CAD build for the part. Positions are in the model's coordinates, mm. A direction names the side the tool comes from. Give positions to 0.01 mm unless a question says otherwise; leave off trailing zeros. Order: outer loops, then holes, each group sorted by start corner. A loop starts at its lowest first (then second) coordinate and runs counter-clockwise, first axis right, second up.
from build123d import *

# Parameters (mm, degrees)
SKETCH1_W            = 18
SKETCH1_H            = 18.5
BOSS_EXTRUDE1_DEPTH  = 3.3
SKETCH2_W            = 18
SKETCH2_H            = 18.5
BOSS_EXTRUDE2_DEPTH  = 0.7
FILLET1_R            = 3
SKETCH3_W            = 13.9
SKETCH3_H            = 14.6
BOSS_EXTRUDE3_DEPTH  = 3.9
SKETCH4_W            = 13.9
SKETCH4_H            = 14.6
SKETCH4_R            = 4.25
BOSS_EXTRUDE4_DEPTH  = 1.5
CHAMFER1_SIZE        = 1
BOSS_EXTRUDE5_DEPTH  = 2
SKETCH6_W            = 0.6
SKETCH6_H            = 6
CUT_EXTRUDE1_DEPTH   = 15.876911642
SKETCH7_W            = 0.7
SKETCH7_H            = 6
CUT_EXTRUDE2_DEPTH   = 14
SKETCH8_W            = 2.65
SKETCH8_H            = 2.4
BOSS_EXTRUDE6_DEPTH  = 0.2
SKETCH9_W            = 2.65
SKETCH9_H            = 2.4
BOSS_EXTRUDE7_DEPTH  = 0.2
CUT_EXTRUDE3_DEPTH   = 18.893085257
CUT_EXTRUDE5_START   = -7.9
CUT_EXTRUDE5_DEPTH   = 7.9
CUT_EXTRUDE7_START   = -4.6
SKETCH12_W           = 0.378675411
SKETCH12_H           = 6.25
CUT_EXTRUDE7_DEPTH   = 4.6
BOSS_EXTRUDE10_DEPTH = 3.3
FILLET2_R            = 2
BOSS_EXTRUDE11_DEPTH = 0.6
SKETCH15_R           = 1.3
CUT_EXTRUDE8_DEPTH   = 18.622783549


with BuildPart() as part:
    # Sketch1 → Boss-Extrude1 (new body)
    with BuildSketch(Plane.XY):
        Rectangle(SKETCH1_W, SKETCH1_H)
        Polygon((-3, -8.25), (-3, -3.25), (-8.2, -3.25), (-8.2, 8.25), (3, 8.25), (3, 3.25), (7.473843231, 3.25), (8.2, 3.25), (8.2, -8.25), align=None, mode=Mode.SUBTRACT)
    extrude(amount=BOSS_EXTRUDE1_DEPTH)

    # Sketch2 → Boss-Extrude2 (add)
    with BuildSketch(Plane.XY.offset(3.3)):
        Rectangle(SKETCH2_W, SKETCH2_H)
        Polygon((-6, 6.5), (3, 6.5), (3, 3.25), (6, 3.25), (6, -6.5), (-3, -6.5), (-3, -3.25), (-6, -3.25), align=None, mode=Mode.SUBTRACT)
    extrude(amount=BOSS_EXTRUDE2_DEPTH)

    # Fillet1
    fillet1_edges = [part.edges().sort_by_distance(p)[0] for p in [
        (-9, 9.25, 2),
        (9, 9.25, 2),
        (9, -9.25, 2),
        (-9, -9.25, 2),
    ]]
    fillet(fillet1_edges, radius=FILLET1_R)

    # Sketch3 → Boss-Extrude3 (add)
    with BuildSketch(Plane.XY.offset(4)):
        Rectangle(SKETCH3_W, SKETCH3_H)
        Polygon((-6, 6.5), (3, 6.5), (3, 3.25), (6, 3.25), (6, -6.5), (-3, -6.5), (-3, -3.25), (-6, -3.25), align=None, mode=Mode.SUBTRACT)
    extrude(amount=BOSS_EXTRUDE3_DEPTH)

    # Sketch4 → Boss-Extrude4 (add)
    with BuildSketch(Plane.XY.offset(7.9)):
        Rectangle(SKETCH4_W, SKETCH4_H)
        Circle(SKETCH4_R, mode=Mode.SUBTRACT)
    extrude(amount=BOSS_EXTRUDE4_DEPTH)

    # Chamfer1
    chamfer1_edges = [part.edges().sort_by_distance(p)[0] for p in [
        (-6.95, 7.3, 6.7),
        (-6.95, -7.3, 6.7),
        (6.95, -7.3, 6.7),
        (6.95, 7.3, 6.7),
        (-6.95, 0, 9.4),
        (0, -7.3, 9.4),
        (6.95, 0, 9.4),
        (0, 7.3, 9.4),
    ]]
    chamfer(chamfer1_edges, length=CHAMFER1_SIZE)

    # Sketch5 → Boss-Extrude5 (add)
    with BuildSketch(Plane.XY.offset(9.4)):
        with BuildLine():
            Line((-2.846728769, 4.470585567), (-2.109207508, 3.689680703))
            ThreePointArc((-2.109207508, 3.689680703), (3.089805898, 2.918150015), (3.563233813, -2.316433637))
            Line((3.563233813, -2.316433637), (4.300755074, -3.097338502))
            ThreePointArc((4.300755074, -3.097338502), (3.853169709, 3.639104725), (-2.846728769, 4.470585567))
        make_face()
        with BuildLine():
            Line((2.846728769, -4.470585567), (2.109207508, -3.689680703))
            ThreePointArc((2.109207508, -3.689680703), (-3.089805898, -2.918150015), (-3.563233813, 2.316433637))
            Line((-3.563233813, 2.316433637), (-4.300755074, 3.097338502))
            ThreePointArc((-4.300755074, 3.097338502), (-3.853169709, -3.639104725), (2.846728769, -4.470585567))
        make_face()
    extrude(amount=BOSS_EXTRUDE5_DEPTH)

    # Sketch6 → Cut-Extrude1 (cut, through all)
    with BuildSketch(Plane.XY.offset(4)):
        with Locations((7.25, 0)):
            Rectangle(SKETCH6_W, SKETCH6_H)
        with Locations((-7.25, 0)):
            Rectangle(SKETCH6_W, SKETCH6_H)
    extrude(amount=-CUT_EXTRUDE1_DEPTH, mode=Mode.SUBTRACT)

    # Sketch7 → Cut-Extrude2 (cut)
    with BuildSketch(Plane(origin=(6.95, 0, 0), x_dir=(0, 0, -1), z_dir=(1, 0, 0))):
        with Locations((-3.65, 0)):
            Rectangle(SKETCH7_W, SKETCH7_H)
    extrude(amount=-CUT_EXTRUDE2_DEPTH, mode=Mode.SUBTRACT)

    # Sketch8 → Boss-Extrude6 (add)
    with BuildSketch(Plane(origin=(6.95, 0, 0), x_dir=(0, 0, -1), z_dir=(1, 0, 0))):
        with Locations((-6.575, 0)):
            Rectangle(SKETCH8_W, SKETCH8_H)
    extrude(amount=BOSS_EXTRUDE6_DEPTH)

    # Sketch9 → Boss-Extrude7 (add)
    with BuildSketch(Plane.ZY.offset(6.95)):
        with Locations((6.575, 0)):
            Rectangle(SKETCH9_W, SKETCH9_H)
    extrude(amount=BOSS_EXTRUDE7_DEPTH)

    # Sketch10 → Cut-Extrude3 (cut, through all)
    with BuildSketch(Plane.XZ.offset(1.2)):
        Polygon((-6.95, 7.9), (-7.15, 5.85), (-7.15, 7.9), align=None)
        Polygon((6.95, 7.9), (7.15, 5.85), (7.15, 7.9), align=None)
    extrude(amount=-CUT_EXTRUDE3_DEPTH, mode=Mode.SUBTRACT)

    # Sketch11 → Cut-Extrude5 (cut)
    with BuildSketch(Plane(origin=(0, 0, 0), x_dir=(-1, 0, 0), z_dir=(0, 0, -1)).offset(CUT_EXTRUDE5_START)):
        with BuildLine():
            Line((-4.578389967, 6.802818924), (-3.862648789, 6.027432648))
            ThreePointArc((-3.862648789, 6.027432648), (-3.439450113, 6.278549428), (-3, 6.5))
            Line((-3, 6.5), (-3, 3.25))
            Line((-3, 3.25), (-6.378675411, 3.25))
            ThreePointArc((-6.378675411, 3.25), (-6.063337952, 3.806039001), (-5.699657401, 4.331732391))
            Line((-5.699657401, 4.331732391), (-6.415398578, 5.107118667))
            ThreePointArc((-6.415398578, 5.107118667), (-5.290584801, 5.731466868), (-4.578389967, 6.802818924))
        make_face()
        with BuildLine():
            Line((4.578389967, -6.802818924), (3.862648789, -6.027432648))
            ThreePointArc((3.862648789, -6.027432648), (3.439450113, -6.278549428), (3, -6.5))
            Line((3, -6.5), (3, -3.25))
            Line((3, -3.25), (6.378675411, -3.25))
            ThreePointArc((6.378675411, -3.25), (6.063337952, -3.806039001), (5.699657401, -4.331732391))
            Line((5.699657401, -4.331732391), (6.415398578, -5.107118667))
            ThreePointArc((6.415398578, -5.107118667), (5.290584801, -5.731466868), (4.578389967, -6.802818924))
        make_face()
    extrude(amount=CUT_EXTRUDE5_DEPTH, mode=Mode.SUBTRACT)

    # Sketch12 → Cut-Extrude7 (cut)
    with BuildSketch(Plane(origin=(0, 0, 3.3), x_dir=(-1, 0, 0), z_dir=(0, 0, -1)).offset(CUT_EXTRUDE7_START)):
        with Locations((-6.189337705, 0.125)):
            Rectangle(SKETCH12_W, SKETCH12_H)
        with Locations((6.189337705, -0.125)):
            Rectangle(SKETCH12_W, SKETCH12_H)
    extrude(amount=CUT_EXTRUDE7_DEPTH, mode=Mode.SUBTRACT)

    # Sketch13 → Boss-Extrude10 (add)
    with BuildSketch(Plane(origin=(0, 0, 0), x_dir=(-1, 0, 0), z_dir=(0, 0, -1))):
        with BuildLine():
            Line((-1.342004098, -8.25), (1.342004098, -8.25))
            ThreePointArc((1.342004098, -8.25), (0, -7.69645725), (-1.342004098, -8.25))
        make_face()
        with BuildLine():
            Line((-1.342004098, 8.25), (1.342004098, 8.25))
            ThreePointArc((1.342004098, 8.25), (0, 7.695), (-1.342004098, 8.25))
        make_face()
    extrude(amount=-BOSS_EXTRUDE10_DEPTH)

    # Fillet2
    fillet2_edges = [part.edges().sort_by_distance(p)[0] for p in [
        (-8.2, 8.25, 1.65),
        (8.2, -8.25, 1.65),
    ]]
    fillet(fillet2_edges, radius=FILLET2_R)

    # Sketch14 → Boss-Extrude11 (add)
    with BuildSketch(Plane(origin=(0, 0, 0), x_dir=(-1, 0, 0), z_dir=(0, 0, -1))):
        with BuildLine():
            Line((-1.871089255, -9.25), (1.871089255, -9.25))
            ThreePointArc((1.871089255, -9.25), (0, -7.69645725), (-1.871089255, -9.25))
        make_face()
        with BuildLine():
            Line((-1.871089255, 9.25), (1.871089255, 9.25))
            ThreePointArc((1.871089255, 9.25), (0, 7.69645725), (-1.871089255, 9.25))
        make_face()
    extrude(amount=BOSS_EXTRUDE11_DEPTH)

    # Sketch15 → Cut-Extrude8 (cut, through all)
    with BuildSketch(Plane(origin=(0, 0, -0.6), x_dir=(-1, 0, 0), z_dir=(0, 0, -1))):
        with Locations((0, 9.6)):
            Circle(SKETCH15_R)
        with Locations((0, -9.6)):
            Circle(SKETCH15_R)
    extrude(amount=-CUT_EXTRUDE8_DEPTH, mode=Mode.SUBTRACT)


solid = part.part
1. Saw through at B-B on y = 1.5. State how many separate pieces and enclosed holes the cut face has, plus the area to 3 significant figures.
2. Pin check, flat tips, straight feed: P1, Ø5.5, axis at x = 3, y = -0.5, coming from the -Z side; P2, Ø0.6, axis at x = 6.5, y = -1.5, coming from the -Z side; P3, Ø0.8, axis at x = -6.5, z = 4.5, coming from the -Y side. Stop position of each tip, or through.
3. Saw through at D-D on y = -4. Give the cut face in (x, z), plus the area to 3 significant figures.
4. Mould opens along X. For faces 4 (the flat face through (5, -7, 3.3)), 5 (the flat face through (-6.27, -6.6, 8.78)), 6 (the cylindrical face through (-7.63, 7.65, 1.67)), 7 (the flat face through (6.44, -0.09, 8.91)) say: released by +X, released by -X, zero draft, split by the parting line, or undercut.
5. 3-axis set-ups, long thin cutter, end or side, ignore diameter. For faces 1 (the flat face through (-6.44, 6.81, 6.23)), 2 (the cylindrical face through (3.923, 3.564, 10.386)), 3 (the flat face through (-4, 8.25, 2)): which of +Z, -Z, +X, -X, +Y, -Y reach the whole face in a straight line?
6. Wall check: line 1 (Y direction, x = 0.25, z = 7); line 2 (X direction, y = 0, z = 8.35); line 3 (Z direction, x = -0.75, y = -5.5). Give the ranges that are in metal, low to high.
7. Saw through at C-C on z = 4.5. Give the cut face in (x, y), plus the area to 3 significant figures.
Reported:
1. separate pieces: 4
1. enclosed holes: 0
1. area: 24.1 mm2
2. P1: stops at z = 7.9
2. P2: stops at z = 4
2. P3: stops at y = -7.15
3. outline: (-9, 0) - (-5.94, 0) - (-5.94, 7.9) - (-1.44, 7.9) - (-1.44, 11.4) - (-3.48, 11.4) - (-3.48, 9.4) - (-5.95, 9.4) - (-6.95, 8.4) - (-6.95, 4) - (-9, 4) - close; (1.44, 7.9) - (6, 7.9) - (6, 3.3) - (8.2, 3.3) - (8.2, 0) - (9, 0) - (9, 4) - (6.95, 4) - (6.95, 8.4) - (5.95, 9.4) - (2.4, 9.4) - (2.4, 11.4) - (1.44, 11.4) - close
3. area: 46.2 mm2
4. face 4: undercut
4. face 5: released by -X
4. face 6: undercut
4. face 7: released by +X
5. face 1: +Z, -X, +Y
5. face 2: +Z
5. face 3: -Z
6. line 1: y = -7.3 to -6.5, 6.5 to 7.3
6. line 2: x = -6.95 to -4.25, 4.25 to 6.95
6. line 3: z = 7.9 to 9.4
7. outline: (-6.95, -6.3) - (-5.95, -7.3) - (5.95, -7.3) - (6.95, -6.3) - (6.95, 6.3) - (5.95, 7.3) - (-5.95, 7.3) - (-6.95, 6.3) - close; hole (-6.42, -5.11) arc R2.72 cw to (-4.58, -6.8) - (-3.86, -6.03) arc R7.16 ccw to (-3, -6.5) - (6, -6.5) - (6, -3) - (6.38, -3) - (6.38, 3.25) arc R7.16 ccw to (5.7, 4.33) - (6.42, 5.11) arc R2.72 cw to (4.58, 6.8) - (3.86, 6.03) arc R7.16 ccw to (3, 6.5) - (-6, 6.5) - (-6, 3) - (-6.38, 3) - (-6.38, -3.25) arc R7.16 ccw to (-5.7, -4.33) - close
7. area: 42.4 mm2
